from build123d import *

# Parameters (mm, degrees)
SKETCH1_W           = 130
SKETCH1_H           = 120
BOSS_EXTRUDE1_DEPTH = 3
CUT_EXTRUDE1_START  = -4
SKETCH2_W           = 20
SKETCH2_H           = 95
CUT_EXTRUDE1_DEPTH  = 5
CUT_EXTRUDE2_START  = -4
SKETCH3_R           = 6
CUT_EXTRUDE2_DEPTH  = 5


with BuildPart() as part:
    # Sketch1 → Boss-Extrude1 (new body)
    with BuildSketch(Plane(origin=(0, 0, 0), x_dir=(1, 0, 0), z_dir=(0, 1, 0))):
        Rectangle(SKETCH1_W, SKETCH1_H)
    extrude(amount=BOSS_EXTRUDE1_DEPTH)

    # Sketch2 → Cut-Extrude1 (cut)
    with BuildSketch(Plane(origin=(0, 3, 0), x_dir=(1, 0, 0), z_dir=(0, 1, 0)).offset(CUT_EXTRUDE1_START)):
        with Locations((-16.25, 0)):
            Rectangle(SKETCH2_W, SKETCH2_H)
    cut_extrude1 = extrude(amount=CUT_EXTRUDE1_DEPTH, mode=Mode.SUBTRACT)

    # Mirror1: Cut-Extrude1 across plane
    add(cut_extrude1.mirror(Plane(origin=(0, 0, 0), x_dir=(0, 0, 1), z_dir=(1, 0, 0))), mode=Mode.SUBTRACT)

    # Sketch3 → Cut-Extrude2 (cut)
    with BuildSketch(Plane(origin=(0, 3, 0), x_dir=(1, 0, 0), z_dir=(0, 1, 0)).offset(CUT_EXTRUDE2_START)):
        with Locations((44.5, 0)):
            Circle(SKETCH3_R)
    cut_extrude2 = extrude(amount=CUT_EXTRUDE2_DEPTH, mode=Mode.SUBTRACT)

    # Mirror2: Cut-Extrude2 across plane
    add(cut_extrude2.mirror(Plane(origin=(0, 0, 0), x_dir=(0, 0, 1), z_dir=(1, 0, 0))), mode=Mode.SUBTRACT)


solid = part.part
For this review, take the finished solid that the model builds, in its own axes (mm). A direction names the side the tool comes from. Round coordinates to 2 decimals unless told otherwise and drop trailing zeros. Loops run counter-clockwise (first coordinate to the right, second up) from the corner with the lowest first, then second, coordinate; pieces in that order, holes last. Notation, with made-up numbers: (-18, 77.5) - (7, 77.5) arc R11 ccw to (7, 96.5) - close; hole circle Ø3 at (51, 79.25). An arc over 180 degrees is marked (long way). Put each result on its own line as item: value. Start each with the question number.
1. Consider section D-D on z = -41. State the section outline as (x, y) points, plus the area to 3 significant figures.
2. Consider section A-A on y = 1.7. State the section outline as (x, z) points, plus the area to 3 significant figures.
3. For faces 4 (the flat face through (65, 1, 1)), 5 (the flat face through (-6.25, 1, 1)), list the 3-axis set-ups (+Z, -Z, +X, -X, +Y, -Y) from which the entire face can be reached by the end or side of a thin tool; tool diameter is ignored.
4. For probe 1 along X at (y, z) = (2.45, -33); probe 2 along Z at (x, y) = (13, 1.6); probe 3 along Z at (x, y) = (-44.5, 2), list the stretches that pass through material, from the lowest coordinate up. Write a range as [from, to].
5. Consider section C-C on z = 0. State the section outline as (x, y) points.
6. Mouldability with a two-part tool opening along Z and no side actions: class faces 1 (the flat face through (-65, 1, 1)), 2 (the flat face through (-26.25, 1, 1)), 3 (the flat face through (-1, 1, 60)) as +Z half, -Z half, draft (parallel to the pull), parting line (faces both ways), or undercut.
7. Consider section B-B on x = -20.5. State the section outline as (y, z) points.
Result sheet:
1. outline: (-65, 0) - (-26.25, 0) - (-26.25, 3) - (-65, 3) - close; (-6.25, 0) - (6.25, 0) - (6.25, 3) - (-6.25, 3) - close; (26.25, 0) - (65, 0) - (65, 3) - (26.25, 3) - close
1. area: 270 mm^2
2. outline: (-65, -60) - (65, -60) - (65, 60) - (-65, 60) - close; hole circle Ø12 at (-44.5, 0); hole (-26.25, -47.5) - (-6.25, -47.5) - (-6.25, 47.5) - (-26.25, 47.5) - close; hole (6.25, -47.5) - (26.25, -47.5) - (26.25, 47.5) - (6.25, 47.5) - close; hole circle Ø12 at (44.5, 0)
2. area: 11,600 mm^2
3. face 4: +Z, -Z, +X, +Y, -Y
3. face 5: +Y, -Y
4. probe 1: [-65, -26.25], [-6.25, 6.25], [26.25, 65]
4. probe 2: [-60, -47.5], [47.5, 60]
4. probe 3: [-60, -6], [6, 60]
5. outline: (-65, 0) - (-50.5, 0) - (-50.5, 3) - (-65, 3) - close; (-38.5, 0) - (-26.25, 0) - (-26.25, 3) - (-38.5, 3) - close; (-6.25, 0) - (6.25, 0) - (6.25, 3) - (-6.25, 3) - close; (26.25, 0) - (38.5, 0) - (38.5, 3) - (26.25, 3) - close; (50.5, 0) - (65, 0) - (65, 3) - (50.5, 3) - close
6. face 1: draft
6. face 2: undercut
6. face 3: +Z half
7. outline: (0, -60) - (3, -60) - (3, -47.5) - (0, -47.5) - close; (0, 47.5) - (3, 47.5) - (3, 60) - (0, 60) - close
